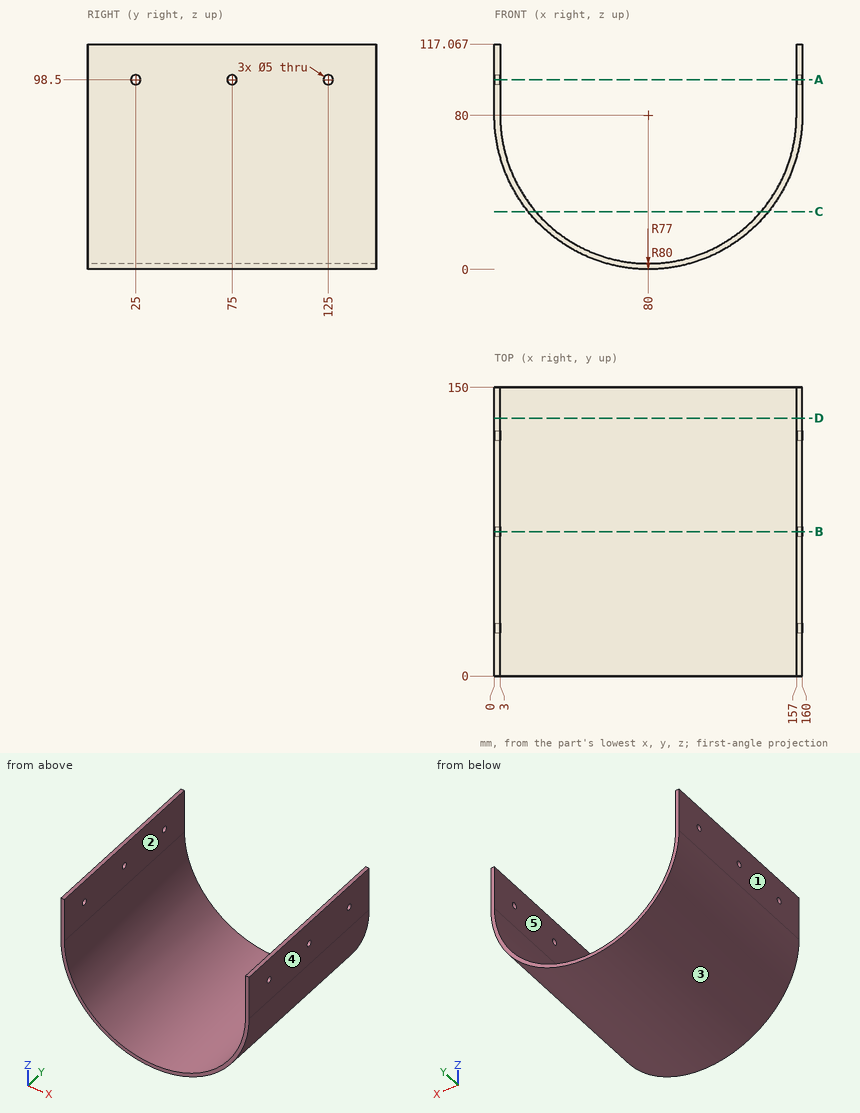
The drawing under review shows one solid part. Ordinate dimensions are in mm from its lowest x, y, z. A direction names the side the tool comes from. Coordinates: 2 decimals unless noted, no trailing zeros. Write each loop counter-clockwise with the first axis right and the second up, starting at its lowest first coordinate (ties: lowest second). Pieces come first, ordered by that corner, then holes. Notation, with made-up numbers: (20.5, 78) - (26.5, 78) arc R24 ccw to (26.5, 90) - close; hole circle Ø7 at (21, 61). An arc over 180 degrees is marked (long way). Put each result on its own line as item: value.
1. For pin 1 (8 mm diameter, centred on y = 97.5, z = 29.5, fed in from -X); pin 2 (1 mm diameter, centred on x = 43, y = 115.5, fed in from +Z); pin 3 (12 mm diameter, centred on x = 82, y = 80, fed in from +Z); pin 4 (3 mm diameter, centred on y = 25, z = 98.5, fed in from +X), all flat-tipped, find the tip position at first contact; note any pin that passes through.
Values found:
pin 1: x = 14.9
pin 2: z = 12.75
pin 3: z = 3.42
pin 4: through
2. Machinability: for the marked faces 4 and 5, which of the approach directions +Z, -Z, +X, -X, +Y, -Y give a long, thin tool a straight path to every point of the face, cutting with its end or side? Answer none if there is none.
Values found:
face 4: +Z, -Z, +X, +Y, -Y
face 5: +Z, +Y, -Y
3. Wall thickness on probe 1 along Y at (x, z) = (1, 98); probe 2 along Y at (x, z) = (1.75, 98.5); probe 3 along X at (y, z) = (12.5, 94): over which ranges is each line inside the solid? List them lowest first.
Values found:
probe 1: 0 to 22.55, 27.45 to 72.55, 77.45 to 122.55, 127.45 to 150
probe 2: 0 to 22.5, 27.5 to 72.5, 77.5 to 122.5, 127.5 to 150
probe 3: 0 to 3, 157 to 160
4. Add section A-A, the plane z = 98.5. Count the separate pieces of the cut face and the enclosed holes in it, then the cut area to 3 significant figures.
Values found:
separate pieces: 8
enclosed holes: 0
area: 810 mm²
5. Add section B-B, the plane y = 75. Give the boundary of the cut face in (x, z).
Values found:
outline: (0, 80) arc R80 ccw to (160, 80) - (160, 96) - (157, 96) - (157, 80) arc R77 cw to (3, 80) - (3, 96) - (0, 96) - close; (0, 101) - (3, 101) - (3, 117.07) - (0, 117.07) - close; (157, 101) - (160, 101) - (160, 117.07) - (157, 117.07) - close
6. Mouldability with a two-part tool opening along X and no side actions: class the marked faces 1, 2 and 3 as released by +X, released by -X, zero draft, split by the parting line, or undercut.
Values found:
face 1: released by -X
face 2: undercut
face 3: split by the parting line
7. Add section C-C, the plane z = 30. Give the boundary of the cut face in (x, y).
Values found:
outline: (17.55, 0) - (21.44, 0) - (21.44, 150) - (17.55, 150) - close; (138.56, 0) - (142.45, 0) - (142.45, 150) - (138.56, 150) - close
8. Add section D-D, the plane y = 134. Give the boundary of the cut face in (x, z).
Values found:
outline: (0, 80) arc R80 ccw to (160, 80) - (160, 117.07) - (157, 117.07) - (157, 80) arc R77 cw to (3, 80) - (3, 117.07) - (0, 117.07) - close
